Read the model definition and answer for the solid it produces. Units are mm, in the model's axes. Face numbers are marked on the shaded views. Give positions to 0.01 mm unless a question says otherwise; leave off trailing zeros. Loops run counter-clockwise (first coordinate to the right, second up) from the corner with the lowest first, then second, coordinate; pieces in that order, holes last. Notation, with made-up numbers: (85, -17.75) - (104, -17.75) arc R26 ccw to (104, 10.25) - close; hole circle Ø8 at (25.5, -31). An arc over 180 degrees is marked (long way). Put each result on its own line as item: value. Start each with the question number.
1. A cutting plane is placed at C-C, the plane z = -2. Determine the outline of the cut face in (x, y).
2. A cutting plane is placed at A-A, the plane y = 25. Determine the outline of the cut face in (x, z).
3. For a pull along X with two mould halves and no side action, classify the marked faces 1, 2 and 3 as released by +X, released by -X, zero draft, split by the parting line, or undercut.
4. Consider L1, parallel to Z at x = -6, y = 18; L2, parallel to X at y = -29.5, z = -3; L3, parallel to Y at x = -13.5, z = 3.25. Determine where each line is inside the solid, lowest interval first. Write a range as from..to.
5. Given pin 1 Ø3 at (x, z) = (6, 0) entering from -Y; pin 2 Ø2 at (x, z) = (-6, 0) entering from +Y, each flat-ended and moving along its own axis, determine where each tip first touches the part or whether it passes through.
6. A cutting plane is placed at B-B, the plane x = 0. Determine the outline of the cut face in (y, z), plus the area to 3 significant figures.
```python
from build123d import *

# Parameters (mm, degrees)
SKETCH1_W                 = 30
SKETCH1_H                 = 66.4
BOSS_EXTRUDE1_DEPTH       = 5
F_6_0MM_DOWEL_HOLE1_D     = 5.9
M3X0_5_TAPPED_HOLE1_D     = 2.5
M3X0_5_TAPPED_HOLE1_DEPTH = 21
M3X0_5_TAPPED_HOLE1_TIP   = 0.751075774
FILLET1_R                 = 10
FILLET2_R                 = 1


with BuildPart() as part:
    # Sketch1 → Boss-Extrude1 (new body, symmetric)
    with BuildSketch(Plane.XY):
        Rectangle(SKETCH1_W, SKETCH1_H)
    extrude(amount=BOSS_EXTRUDE1_DEPTH, both=True)

    # Ø6.0mm Dowel Hole1 (through all)
    with Locations(Plane.XY.offset(5)):
        with Locations((0, -27.2)):
            Hole(F_6_0MM_DOWEL_HOLE1_D / 2)

    # M3x0.5 Tapped Hole1
    with Locations(Plane(origin=(0, 33.2, 0), x_dir=(1, 0, 0), z_dir=(0, 1, 0))):
        with Locations((-6, 0), (6, 0)):
            Hole(M3X0_5_TAPPED_HOLE1_D / 2, depth=M3X0_5_TAPPED_HOLE1_DEPTH)
            with Locations((0, 0, -(M3X0_5_TAPPED_HOLE1_DEPTH + M3X0_5_TAPPED_HOLE1_TIP / 2))):  # 118° drill point
                Cone(0, M3X0_5_TAPPED_HOLE1_D / 2, M3X0_5_TAPPED_HOLE1_TIP, mode=Mode.SUBTRACT)

    # Fillet1
    fillet1_edges = [part.edges().sort_by_distance(p)[0] for p in [
        (15, -33.2, 0),
        (-15, -33.2, 0),
    ]]
    fillet(fillet1_edges, radius=FILLET1_R)

    # Fillet2
    fillet2_edges = [part.edges().sort_by_distance(p)[0] for p in [
        (15, 5, 5),
        (0, -33.2, -5),
        (0, -33.2, 5),
        (12.071067812, -30.271067812, -5),
        (-12.071067812, -30.271067812, -5),
        (12.071067812, -30.271067812, 5),
        (-12.071067812, -30.271067812, 5),
        (-15, 5, 5),
        (15, 5, -5),
        (-15, 5, -5),
    ]]
    fillet(fillet2_edges, radius=FILLET2_R)


solid = part.part
```
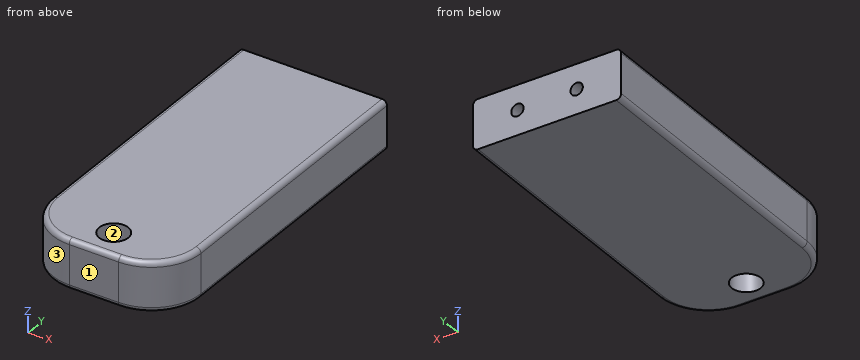
Return value:
1. outline: (-15, -23.2) arc R10 ccw to (-5, -33.2) - (5, -33.2) arc R10 ccw to (15, -23.2) - (15, 33.2) - (-15, 33.2) - close; hole circle Ø5.9 at (0, -27.2)
2. outline: (-15, -4) arc R1 ccw to (-14, -5) - (14, -5) arc R1 ccw to (15, -4) - (15, 4) arc R1 ccw to (14, 5) - (-14, 5) arc R1 ccw to (-15, 4) - close; hole circle Ø2.5 at (-6, 0); hole circle Ø2.5 at (6, 0)
3. face 1: zero draft
3. face 2: undercut
3. face 3: released by -X
4. L1: z = -5..-1.25, 1.25..5
4. L2: x = -12.77..-1.85, 1.85..12.77
4. L3: y = -28.47..33.2
5. pin 1: stops at y = -33.2
5. pin 2: stops at y = 12.05
6. outline: (-33.2, -4) arc R1 ccw to (-32.2, -5) - (-30.15, -5) - (-30.15, 5) - (-32.2, 5) arc R1 ccw to (-33.2, 4) - close; (-24.25, -5) - (33.2, -5) - (33.2, 5) - (-24.25, 5) - close
6. area: 605 mm2
